The model under review builds one solid part; all positions refer to its coordinate system, in mm. A direction names the side the tool comes from. Give positions to 0.01 mm unless a question says otherwise; leave off trailing zeros. Order: outer loops, then holes, each group sorted by start corner. A loop starts at its lowest first (then second) coordinate and runs counter-clockwise, first axis right, second up. Notation, with made-up numbers: (-17, -29.75) - (19, -29.75) arc R31 ccw to (19, -4.75) - close; hole circle Ø6 at (35, 29). An arc over 180 degrees is marked (long way). Answer as CSV lines item,"result". Start each with the question number.
from build123d import *

# Parameters (mm, degrees)
SKETCH_1_W          = 37.5
SKETCH_1_H          = 22.5
EXTRUDE_2_DEPTH     = 4
SKETCH_2_W          = 15
SKETCH_2_H          = 10
EXTRUDE_3_DEPTH     = 18.5
EXTRUDE_4_DEPTH     = 15
EXTRUDE_5_DEPTH     = 8.66025404
SKETCH_5_R          = 1.7
CUT_EXTRUDE_1_DEPTH = 10
FILLET_1_R          = 15
FILLET_3_R          = 5
SKETCH_9_R          = 1.8
CUT_EXTRUDE_2_DEPTH = 4
FILLET_5_R          = 10
RIB_10_REACH        = 84.489
SKETCH_16_WALL_W    = 186.275176358
SKETCH_16_WALL_H    = 4
RIB_START           = -4
RIB_11_DEPTH        = 4
FILLET_6_R          = 2


# Read off the part's stored shape, not the designer's step: 筋11
with BuildPart() as part:
    # 草图1 → 凸台-拉伸2 (new body)
    with BuildSketch(Plane(origin=(0, 0, 0), x_dir=(1, 0, 0), z_dir=(0, 1, 0))):
        with Locations((18.75, 11.25)):
            Rectangle(SKETCH_1_W, SKETCH_1_H)
    extrude(amount=EXTRUDE_2_DEPTH)

    # 草图2 → 凸台-拉伸3 (add)
    with BuildSketch(Plane(origin=(0, 4, 0), x_dir=(1, 0, 0), z_dir=(0, 1, 0))):
        with Locations((18.75, 11.25)):
            Rectangle(SKETCH_2_W, SKETCH_2_H)
    extrude(amount=EXTRUDE_3_DEPTH)

    # 草图3 → 凸台-拉伸4 (add)
    with BuildSketch(Plane(origin=(26.25, 0, 0), x_dir=(0, 0, -1), z_dir=(1, 0, 0))):
        Polygon((6.25, 22.5), (-17.75, 64.069219382), (-10.25, 68.399346401), (16.25, 22.5), align=None)
    extrude(amount=-EXTRUDE_4_DEPTH)

    # 草图4 → 凸台-拉伸5 (add)
    with BuildSketch(Plane(origin=(0, 8.331329387, -14.430285793), x_dir=(1, 0, 0), z_dir=(0, -0.5000000000000041, 0.8660254037844363))):
        with BuildLine():
            Line((26.25, 64.360571585), (11.25, 64.360571585))
            ThreePointArc((11.25, 64.360571585), (18.75, 71.860571585), (26.25, 64.360571585))
        make_face()
    extrude(amount=-EXTRUDE_5_DEPTH)

    # 草图5 → 切除-拉伸1 (cut)
    with BuildSketch(Plane(origin=(0, 8.331329387, -14.430285793), x_dir=(1, 0, 0), z_dir=(0, -0.5000000000000041, 0.8660254037844363))):
        with Locations(Location((18.75, 64.360571585, 0), (0, 0, 270))):
            Circle(SKETCH_5_R)
        with Locations(Location((18.75, 27.360571585, 0), (0, 0, 270))):
            Circle(SKETCH_5_R)
    extrude(amount=-CUT_EXTRUDE_1_DEPTH, mode=Mode.SUBTRACT)

    # 圆角1
    fillet_1_edges = [part.edges().sort_by_distance(p)[0] for p in [
        (18.75, 22.5, -6.25),
    ]]
    fillet(fillet_1_edges, radius=FILLET_1_R)

    # 圆角3
    fillet_3_edges = [part.edges().sort_by_distance(p)[0] for p in [
        (0, 2, -22.5),
        (37.5, 2, -22.5),
        (37.5, 2, 0),
        (0, 2, 0),
    ]]
    fillet(fillet_3_edges, radius=FILLET_3_R)

    # 草图9 → 切除-拉伸2 (cut)
    with BuildSketch(Plane(origin=(0, 4, 0), x_dir=(1, 0, 0), z_dir=(0, 1, 0))):
        with Locations(Location((5, 17.5, 0), (0, 0, 270))):
            Circle(SKETCH_9_R)
        with Locations(Location((32.5, 17.5, 0), (0, 0, 90))):
            Circle(SKETCH_9_R)
        with Locations(Location((32.5, 5, 0), (0, 0, 270))):
            Circle(SKETCH_9_R)
        with Locations(Location((5, 5, 0), (0, 0, 90))):
            Circle(SKETCH_9_R)
    extrude(amount=-CUT_EXTRUDE_2_DEPTH, mode=Mode.SUBTRACT)

    # 圆角5
    fillet_5_edges = [part.edges().sort_by_distance(p)[0] for p in [
        (18.75, 22.5, -16.25),
    ]]
    fillet(fillet_5_edges, radius=FILLET_5_R)

    # 草图16 wall → 筋10 (add, up to next)
    with BuildSketch(Plane(origin=(26.25, 13.079426042, -19.236382193), x_dir=(0, 0.941051653324, 0.33826289447), z_dir=(0, -0.33826289447, 0.941051653324)), mode=Mode.PRIVATE) as rib_10_sk1:
        with Locations((0, 2)):
            Rectangle(SKETCH_16_WALL_W, SKETCH_16_WALL_H)
    rib_10_tool1 = extrude(rib_10_sk1.sketch, amount=RIB_10_REACH, mode=Mode.PRIVATE) - part.part
    add(rib_10_tool1.solids().sort_by_distance((26.25, 13.079426042, -19.236382193))[0])

    # 筋11 outline → 筋11 (add)
    with BuildSketch(Plane.ZY.offset(-11.25).offset(RIB_START)):
        with BuildLine():
            Line((-15.98478303, 22.108301633), (-22.5, 4))
            Line((-22.5, 4), (-16.25, 4))
            Line((-16.25, 4), (-16.25, 19.820508076))
            ThreePointArc((-16.25, 19.820508076), (-16.183474475, 20.972065652), (-15.98478303, 22.108301633))
        make_face()
    extrude(amount=RIB_11_DEPTH)

    # 圆角6
    # the kernel refuses this fillet: 2 mm, written as the material it takes off along each edge
    with BuildSketch(Plane(origin=(11.25, 68.399346401, 10.25), x_dir=(1.7763568394002473e-15, -0.5000000000000042, 0.8660254037844363), z_dir=(0, -0.8660254037844363, -0.5000000000000042)), Plane(origin=(26.25, 68.399346401, 10.25), x_dir=(-1, 0, 0), z_dir=(0, -0.8660254037844363, -0.5000000000000042))) as fillet_6_piece_1:
        with BuildLine():
            CenterArc((FILLET_6_R, -FILLET_6_R), FILLET_6_R, 90, 90)
            Line((0, -FILLET_6_R), (-FILLET_6_R * 0.02, -FILLET_6_R))
            Line((-FILLET_6_R * 0.02, -FILLET_6_R), (-FILLET_6_R * 0.02, FILLET_6_R * 0.02))
            Line((-FILLET_6_R * 0.02, FILLET_6_R * 0.02), (FILLET_6_R, FILLET_6_R * 0.02))
            Line((FILLET_6_R, FILLET_6_R * 0.02), (FILLET_6_R, 0))
        make_face()
    extrude(amount=62.320508076, mode=Mode.SUBTRACT)
    with BuildSketch(Plane(origin=(18.75, 68.399346402, 10.249999998), x_dir=(-1, 0, 0), z_dir=(0, -0.8660254037844363, -0.5000000000000041))) as fillet_6_piece_2:
        with BuildLine():
            CenterArc((7.5 - FILLET_6_R, -FILLET_6_R * 1.00000000108), FILLET_6_R, 360, 90)
            Line((7.5, -FILLET_6_R * 1.00000000108), (7.5 + FILLET_6_R * 0.02, -FILLET_6_R * 1.00000000108))
            Line((7.5 + FILLET_6_R * 0.02, -FILLET_6_R * 1.00000000108), (7.5 + FILLET_6_R * 0.02, FILLET_6_R * 0.02))
            Line((7.5 + FILLET_6_R * 0.02, FILLET_6_R * 0.02), (7.5 - FILLET_6_R, FILLET_6_R * 0.0199999989222))
            Line((7.5 - FILLET_6_R, FILLET_6_R * 0.0199999989222), (7.5 - FILLET_6_R, -FILLET_6_R * 1.07782831552e-09))
        make_face()
    revolve(axis=Axis((18.75, 68.399346402, 10.249999998), (0, 0.5000000000000041, -0.8660254037844363)), revolution_arc=180, mode=Mode.SUBTRACT)


solid = part.part
Item 1: For line 1 along X through (y, z) = (2.3, -17.5); line 2 along X through (y, z) = (6, -9.5); line 3 along Y through (x, z) = (26.5, -19), list the stretches that pass through material, from the lowest coordinate up.
Item 2: Mouldability with a two-part tool opening along X and no side actions: class faces 6 (the face through (3.243, 2.028, -17.89)), 7 (the face through (18.59, 72.2, 18.66)), 8 (the face through (18.855, 22.416, -5.725)) as released by +X, released by -X, zero draft, split by the parting line, or undercut.
Item 3: Take a section at A-A on x = 6. Write out the cut boundary in (y, z).
Item 4: Clearance check with flat-ended pins moving along their axes: pin 1 (20 mm diameter, centred on y = 46.5, z = -8.5, fed in from -X); pin 2 (1.9 mm diameter, centred on x = 17.5, z = -19, fed in from +Y); pin 3 (1.2 mm diameter, centred on x = 24.5, y = 3, fed in from +Z). State where each tip first meets the part, or that it passes through.
Item 5: Machinability: for faces 1 (the face through (19, 2, 0)), 2 (the face through (13.278, 13.181, -19.197)), 3 (the face through (11.82, 41.65, -4.5)), 4 (the face through (26.25, 34, -2)), 5 (the face through (22.25, 10, -19)), which of the approach directions +Z, -Z, +X, -X, +Y, -Y give a long, thin tool a straight path to every point of the face, cutting with its end or side? Answer none if there is none.
Data:
1,line 1,"x = 0 to 3.2, 6.8 to 30.7, 34.3 to 37.5"
1,line 2,"x = 11.25 to 26.25"
1,line 3,"y = 0 to 4"
2,face 6,"undercut"
2,face 7,"split by the parting line"
2,face 8,"zero draft"
3,outline,"(0, -22.5) - (4, -22.5) - (4, -19) - (0, -19) - close; (0, -16) - (4, -16) - (4, -6.5) - (0, -6.5) - close; (0, -3.5) - (4, -3.5) - (4, 0) - (0, 0) - close"
4,pin 1,"stops at x = 11.25"
4,pin 2,"stops at y = 4"
4,pin 3,"stops at z = 0"
5,face 1,"+Z, +X, -X, -Y"
5,face 2,"-Z, +X, -X, +Y"
5,face 3,"-Z, -X, +Y"
5,face 4,"+Z, -Z, +X, +Y"
5,face 5,"-Z, +Y"
